```python
from build123d import *

# Parameters (mm, degrees)
F0_R     = 14.2875
F1_DEPTH = 25.4


with BuildPart() as f1:
    # F0 (on Right) → F1 (new body)
    with BuildSketch(Plane.YZ):
        with BuildLine():
            Line((161.028833, 175.012099), (14.85964, 175.012099))
            ThreePointArc((14.85964, 175.012099), (9.020452, 171.157371), (10.270549, 164.273164))
            Line((10.270549, 164.273164), (156.439742, 11.437965))
            ThreePointArc((156.439742, 11.437965), (163.393338, 9.933546), (167.378833, 15.8269))
            Line((167.378833, 15.8269), (167.378833, 168.662099))
            ThreePointArc((167.378833, 168.662099), (165.518961, 173.152227), (161.028833, 175.012099))
        make_face()
        with Locations((148.328833, 44.45)):
            Circle(F0_R, mode=Mode.SUBTRACT)
        with Locations((44.45, 155.962099)):
            Circle(F0_R, mode=Mode.SUBTRACT)
        with Locations((148.328833, 155.962099)):
            Circle(F0_R, mode=Mode.SUBTRACT)
    extrude(amount=F1_DEPTH)


solid = f1.part
```
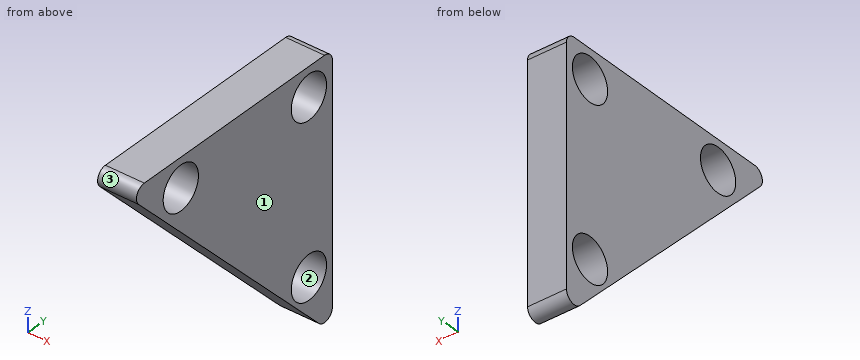
For this review, take the finished solid that the model builds, in its own axes (mm). Face numbers are marked on the shaded views. Round coordinates to 2 decimals unless told otherwise and drop trailing zeros. Write each loop counter-clockwise with the first axis right and the second up, starting at its lowest first coordinate (ties: lowest second). Pieces come first, ordered by that corner, then holes. Notation, with made-up numbers: (57.5, -13.5) - (76.5, -13.5) arc R3 ccw to (76.5, -8.5) - close; hole circle Ø2 at (72, 9). An arc over 180 degrees is marked (long way). Put each result on its own line as item: value.
Q1. We need section B-B (x = 17.5). Count the separate pieces of the cut face and the enclosed holes in it, and give its area (3 significant figures).
Solved:
separate pieces: 1
enclosed holes: 3
area: 12,600 mm2
Q2. Insertion check: pin 1 Ø5 at (x, y) = (17, 82) entering from -Z; pin 2 Ø12 at (x, y) = (3, 85.5) entering from -Z; pin 3 Ø8 at (x, z) = (14, 138.5) entering from -Y; pin 4 Ø1 at (y, z) = (58.5, 158) entering from +X. Each pin has a flat end and moves straight along its axis. Give the tip position at first contact, or say it passes through.
Solved:
pin 1: stops at z = 86.66
pin 2: stops at z = 79.34
pin 3: stops at y = 31.09
pin 4: stops at x = 25.4
Q3. We need section A-A (z = 50.5). Give the boundary of the cut face in (x, y), and give its area (3 significant figures).
Solved:
outline: (0, 119.08) - (25.4, 119.08) - (25.4, 135.39) - (0, 135.39) - close; (0, 161.27) - (25.4, 161.27) - (25.4, 167.38) - (0, 167.38) - close
area: 569 mm2
Q4. We need section D-D (z = 146). Give the boundary of the cut face in (x, y), and give its area (3 significant figures).
Solved:
outline: (0, 27.75) - (25.4, 27.75) - (25.4, 34.21) - (0, 34.21) - close; (0, 54.69) - (25.4, 54.69) - (25.4, 138.09) - (0, 138.09) - close; (0, 158.57) - (25.4, 158.57) - (25.4, 167.38) - (0, 167.38) - close
area: 2,510 mm2
Q5. Mouldability with a two-part tool opening along Y and no side actions: class the marked faces 1, 2 and 3 as released by +Y, released by -Y, zero draft, split by the parting line, or undercut.
Solved:
face 1: zero draft
face 2: undercut
face 3: released by -Y
Q6. Wall thickness on probe 1 along Z at (x, y) = (13.5, 157.5); probe 2 along Z at (x, y) = (7.75, 151); probe 3 along Z at (x, y) = (13.75, 44.45): over which ranges is each line inside the solid? List them lowest first.
Solved:
probe 1: z = 10.55 to 33.49, 55.41 to 145.01, 166.92 to 175.01
probe 2: z = 17.13 to 30.41, 58.49 to 141.93, 170 to 175.01
probe 3: z = 128.53 to 141.67, 170.25 to 175.01
Q7. We need section C-C (y = 44.45). Give the boundary of the cut face in (x, z).
Solved:
outline: (0, 128.53) - (25.4, 128.53) - (25.4, 141.67) - (0, 141.67) - close; (0, 170.25) - (25.4, 170.25) - (25.4, 175.01) - (0, 175.01) - close
